The figure shows three views and two pictorial views of one solid part (mm, origin at its lowest corner). Answer the questions. A direction names the side the tool comes from. Round coordinates to 2 decimals unless told otherwise and drop trailing zeros. Order: outer loops, then holes, each group sorted by start corner. A loop starts at its lowest first (then second) coordinate and runs counter-clockwise, first axis right, second up. Notation, with made-up numbers: (41.25, -15) -> (64.25, -15) arc R17 cw to (64.25, 18) -> close; hole circle Ø1 at (-28.75, 0.5). An arc over 180 degrees is marked (long way). One line per item, written item: value. Start each with the question number.
1. Flat-ended cylindrical pins translate along their axes: pin 1 Ø5 at (x, y) = (134.5, 5.5) entering from -Z; pin 2 Ø5 at (x, y) = (33.5, 7.5) entering from +Z; pin 3 Ø12 at (x, z) = (67, 15.5) entering from +Y. Find the tip coordinate at first contact, or state that the pin passes through.
2. Section A-A (z = 10) is taken. Give the vertices of the cut face in (x, y).
3. For the marked faces 1 and 2, determine the directions among +Z, -Z, +X, -X, +Y, -Y from which every point of the face is accessible in a straight line to the end or side of a thin tool.
4. Section C-C (x = 42.5) is taken. Give the vertices of the cut face in (y, z), then the cut area to 3 significant figures.
5. Consider line 1 (Y direction, x = 38, z = 10.5); line 2 (X direction, y = 3, z = 15.75); line 3 (Y direction, x = 49.5, z = 14.5). Determine where each line is inside the solid, lowest interval first.
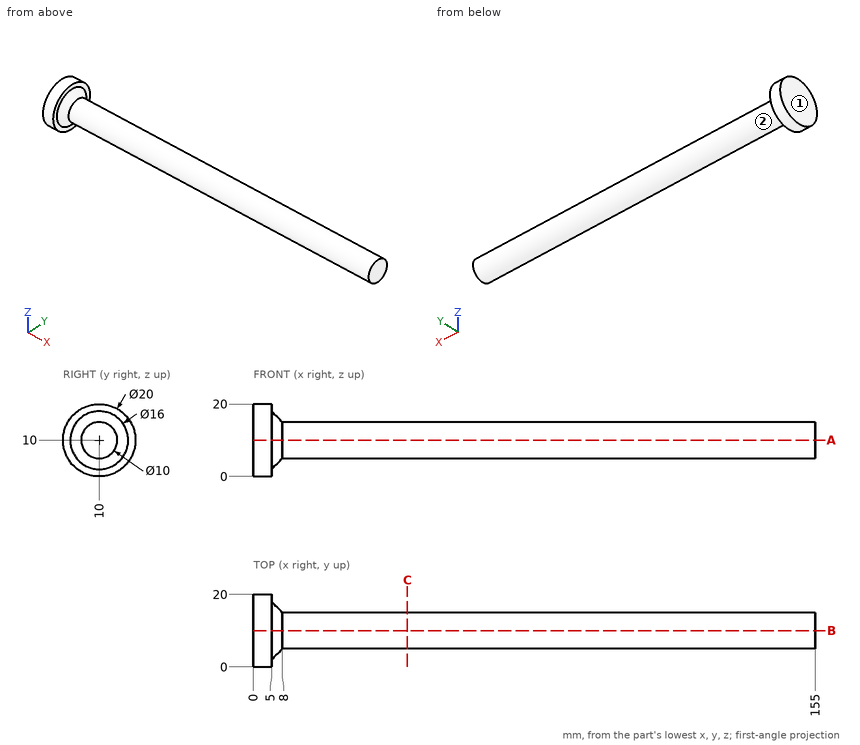
Answer:
1. pin 1: z = 5.42
1. pin 2: z = 15
1. pin 3: y = 15
2. outline: (0, 0) -> (5, 0) -> (5, 2) -> (8, 5) -> (155, 5) -> (155, 15) -> (8, 15) -> (5, 18) -> (5, 20) -> (0, 20) -> close
3. face 1: +Z, -Z, -X, +Y, -Y
3. face 2: +X
4. outline: circle Ø10 at (10, 10)
4. area: 78.5 mm^2
5. line 1: 5.03 to 14.97
5. line 2: 0 to 5
5. line 3: 7.82 to 12.18
